Verification items for this drawing (mm, ordinates from the low corner). A direction names the side the tool comes from. Coordinates: 2 decimals unless noted, no trailing zeros. Order: outer loops, then holes, each group sorted by start corner. A loop starts at its lowest first (then second) coordinate and runs counter-clockwise, first axis right, second up.
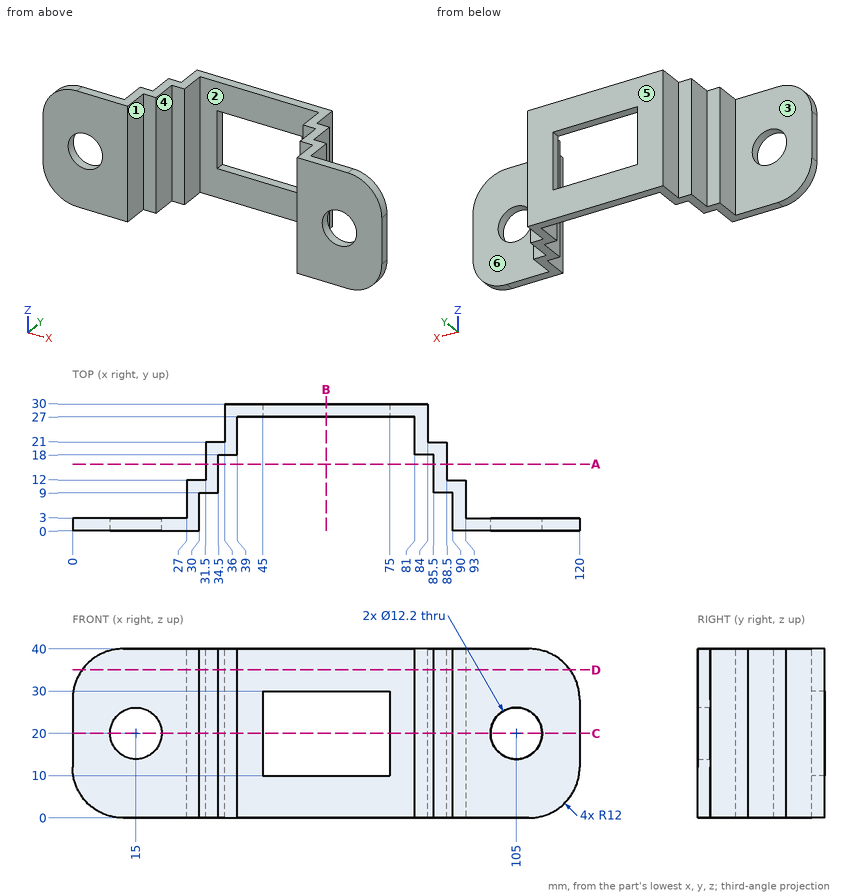
Item 1: Sectioned sample at C-C (z = 20). Give the number of separate pieces and of enclosed holes in the cut face, and give its area (3 significant figures).
Item 2: Thickness scan on line 1 along X through (y, z) = (1.5, 20); line 2 along X through (y, z) = (13.25, 11); line 3 along X through (y, z) = (8.75, 35). Record the ranges inside material, lowest first.
Item 3: Release check for a two-part mould opening along X. For the marked faces 1, 2 and 3 record: pulls with the +X half, pulls with the -X half, needs draft (parallel to the pull), parting line crosses it, or undercut.
Item 4: Depth check by flat-ended pin: P1, Ø2.5, axis at y = 23.5, z = 23, coming from the +X side; P2, Ø1.3, axis at x = 90, z = 23, coming from the +Y side; P3, Ø6, axis at x = 81, z = 32, coming from the -Y side; P4, Ø8, axis at x = 68.5, y = 20.5, coming from the -Z side. Enter the tip coordinate at first touch or a pass-through.
Item 5: Sectioned sample at B-B (x = 60). Record the cut outline in (y, z), and give its area (3 significant figures).
Item 6: Sectioned sample at A-A (y = 15.75). Record the cut outline in (x, z).
Item 7: Sectioned sample at D-D (z = 35). Record the cut outline in (x, y).
Item 8: Tool access check on the marked faces 4, 5 and 6. Record the directions out of +Z, -Z, +X, -X, +Y, -Y that give a thin tool (end or side, any length) a straight path to the whole face; none if there is none.
Geometry check:
1. separate pieces: 4
1. enclosed holes: 0
1. area: 359 mm2
2. line 1: x = 0 to 8.9, 21.1 to 30, 90 to 98.9, 111.1 to 120
2. line 2: x = 31.5 to 34.5, 85.5 to 88.5
2. line 3: x = 27 to 30, 90 to 93
3. face 1: undercut
3. face 2: undercut
3. face 3: needs draft
4. P1: stops at x = 84
4. P2: stops at y = 12
4. P3: stops at y = 18
4. P4: passes through
5. outline: (27, 0) - (30, 0) - (30, 10) - (27, 10) - close; (27, 30) - (30, 30) - (30, 40) - (27, 40) - close
5. area: 60.0 mm2
6. outline: (31.5, 0) - (34.5, 0) - (34.5, 40) - (31.5, 40) - close; (85.5, 0) - (88.5, 0) - (88.5, 40) - (85.5, 40) - close
7. outline: (2.25, 0) - (30, 0) - (30, 9) - (34.5, 9) - (34.5, 18) - (39, 18) - (39, 27) - (81, 27) - (81, 18) - (85.5, 18) - (85.5, 9) - (90, 9) - (90, 0) - (117.75, 0) - (117.75, 3) - (93, 3) - (93, 12) - (88.5, 12) - (88.5, 21) - (84, 21) - (84, 30) - (36, 30) - (36, 21) - (31.5, 21) - (31.5, 12) - (27, 12) - (27, 3) - (2.25, 3) - close
8. face 4: +Z, -Z, -Y
8. face 5: +Z, -Z, +X, -X, +Y
8. face 6: +Z, -Z, +X, +Y
